Part print with two shaded views. Sizes in mm from the minimum x, y, z corner. A direction names the side the tool comes from. Give positions to 0.01 mm unless a question says otherwise; leave off trailing zeros. Write each loop counter-clockwise with the first axis right and the second up, starting at its lowest first coordinate (ties: lowest second). Pieces come first, ordered by that corner, then holes.
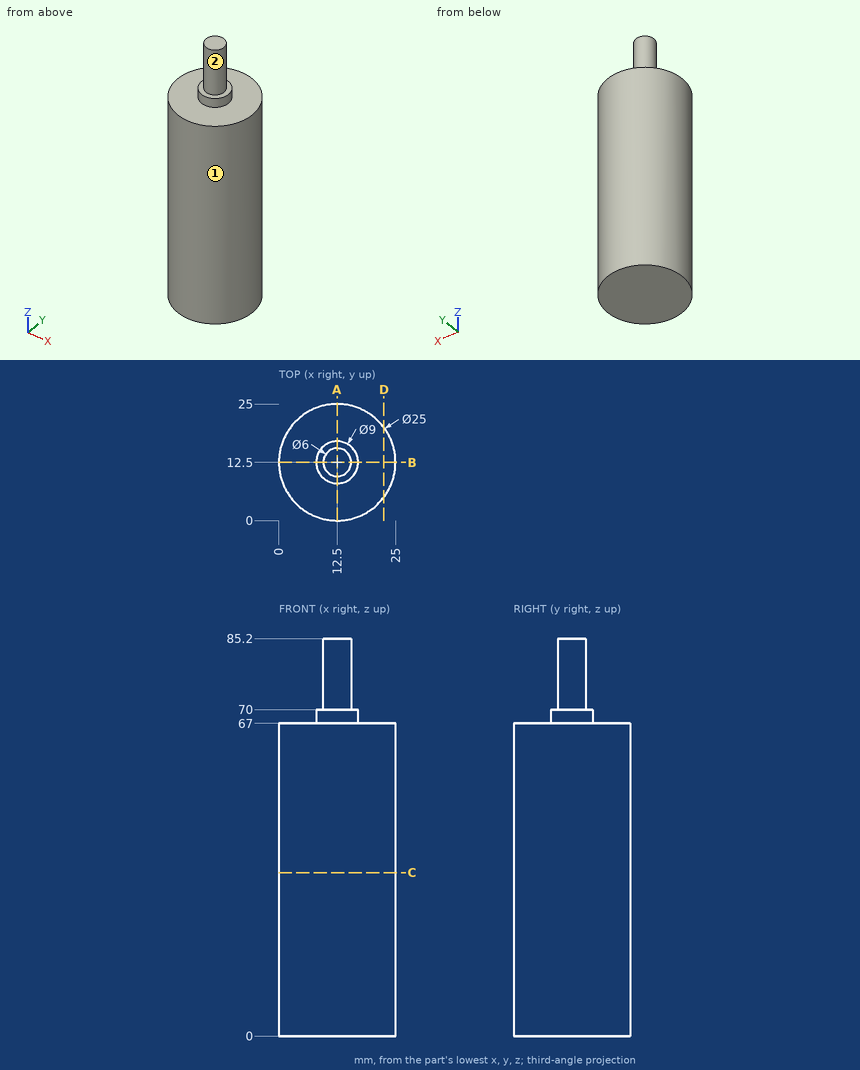
1) Wall check: L1, parallel to Z at x = 6.25, y = 18; L2, parallel to Y at x = 7.25, z = 18; L3, parallel to Y at x = 13.25, z = 80. Give the ranges that are in metal, low to high.
Answers follow:
L1: z = 0 to 67
L2: y = 1.16 to 23.84
L3: y = 9.6 to 15.4
2) Saw through at A-A, the plane x = 12.5. Write the cut outline in (y, z).
Answers follow:
outline: (0, 0) - (25, 0) - (25, 67) - (17, 67) - (17, 70) - (15.5, 70) - (15.5, 85.2) - (9.5, 85.2) - (9.5, 70) - (8, 70) - (8, 67) - (0, 67) - close
3) Saw through at D-D, the plane x = 22.5. Write the cut outline in (y, z).
Answers follow:
outline: (5, 0) - (20, 0) - (20, 67) - (5, 67) - close
4) Pin check, flat tips, straight feed: pin 1 Ø1 at (x, z) = (4, 38.5) entering from -Y; pin 2 Ø4 at (y, z) = (21.5, 21) entering from -X; pin 3 Ø2 at (x, z) = (16, 67) entering from +Y. Stop position of each tip, or through.
Answers follow:
pin 1: stops at y = 2.9
pin 2: stops at x = 2.14
pin 3: stops at y = 24.75
5) 3-axis set-ups, long thin cutter, end or side, ignore diameter. For the marked faces 1 and 2: which of +Z, -Z, +X, -X, +Y, -Y reach the whole face in a straight line?
Answers follow:
face 1: +Z, -Z
face 2: +Z
6) Saw through at C-C, the plane z = 35. Write the cut outline in (x, y).
Answers follow:
outline: circle Ø25 at (12.5, 12.5)
